Read the model definition and answer for the solid it produces. Units are mm, in the model's axes. Face numbers are marked on the shaded views. A direction names the side the tool comes from. Give positions to 0.01 mm unless a question says otherwise; leave off trailing zeros. Order: outer loops, then holes, each group sorted by start corner. A loop starts at its lowest first (then second) coordinate and runs counter-clockwise, first axis right, second up. Notation, with made-up numbers: (29.25, 23) - (33.25, 23) arc R33 ccw to (33.25, 60) - close; hole circle Ø5 at (-1.5, 16). An arc over 180 degrees is marked (long way). Write each question's results on one line, items separated by ' | '. Start each with the question number.
Q1. Find section D-D on x = -10.5. Give the vertices of the cut face in (y, z), and give its area (3 significant figures).
Q2. Find section A-A on x = 4.75. Give the vertices of the cut face in (y, z), and give its area (3 significant figures).
Q3. Find section B-B on y = 1.15. Give the vertices of the cut face in (x, z), and give its area (3 significant figures).
Q4. Find the intervals of material crossed by line 1 along X through (y, z) = (1.1, 11); line 2 along X through (y, z) = (2.6, 8.5); line 3 along X through (y, z) = (0.3, 1), in increasing order. Write a range as from..to.
Q5. A tool of negligible diameter and unlimited length cuts with its end or side. For the marked faces 4, 5 and 6, from which of +Z, -Z, +X, -X, +Y, -Y can it reach the whole face along a straight path? Write none if from no direction.
Q6. Find section C-C on z = 3.25. Give the vertices of the cut face in (x, y), and give its area (3 significant figures).
Q7. Flat-ended cylindrical pins translate along their axes: P1, Ø1.2, axis at x = 9.5, z = 0, coming from the +Y side; P2, Ø3.5, axis at x = 9.9, z = 0, coming from the -Y side; P3, Ø0.9, axis at y = 1.5, z = -10, coming from the -X side; P4, Ø3, axis at x = -9.9, z = 0, coming from the +Y side. Find the tip coordinate at first contact, or state that the pin passes through.
Q8. For a pull along X with two mould halves and no side action, classify the marked faces 1, 2 and 3 as +X half, -X half, draft (parallel to the pull), parting line (faces both ways), or undercut.
from build123d import *

# Parameters (mm, degrees)
EXTRUDE_1_DEPTH          = 3
SKETCH_2_R               = 1.25
CUT_EXTRUDE_1_DEPTH      = 18.930421077
CUT_EXTRUDE_START        = -3
SKETCH_2_3_R             = 2
CUT_EXTRUDE_2_DEPTH      = 1.5
PATTERN_CIRCULAR_1_COUNT = 4


with BuildPart() as part:
    # 草图1 → 凸台-拉伸1 (new body)
    with BuildSketch(Plane(origin=(0, 0, 0), x_dir=(1, 0, 0), z_dir=(0, 1, 0))):
        with BuildLine():
            ThreePointArc((0, 6.2), (4.384062043, 4.384062043), (6.2, 0))
            Line((6.2, 0), (6.2, 6.2))
            Line((6.2, 6.2), (0, 6.2))
        make_face()
        with BuildLine():
            Line((-6.2, 6.2), (-6.2, 1.3e-08))
            ThreePointArc((-6.2, 1.3e-08), (-4.384062039, 4.384062048), (0, 6.2))
            Line((0, 6.2), (-6.2, 6.2))
        make_face()
        with BuildLine():
            Line((-6.2, 1.3e-08), (-6.2, -6.2))
            Line((-6.2, -6.2), (0, -6.2))
            ThreePointArc((0, -6.2), (-4.384062048, -4.384062039), (-6.2, 1.3e-08))
        make_face()
        with BuildLine():
            ThreePointArc((6.2, 0), (4.384062043, -4.384062043), (0, -6.2))
            Line((0, -6.2), (6.2, -6.2))
            Line((6.2, -6.2), (6.2, 0))
        make_face()
        Polygon((0, -6.2), (-6.2, -6.2), (-6.2, -12.5), (6.2, -12.5), (6.2, -6.2), align=None)
        Polygon((6.2, 0), (6.2, -6.2), (12.5, -6.2), (12.5, 6.2), (6.2, 6.2), align=None)
        Polygon((-6.2, 12.5), (-6.2, 6.2), (0, 6.2), (6.2, 6.2), (6.2, 12.5), align=None)
        Polygon((-12.5, 6.2), (-12.5, -6.2), (-6.2, -6.2), (-6.2, 1.3e-08), (-6.2, 6.2), align=None)
    extrude(amount=EXTRUDE_1_DEPTH)

    # 草图2 → 切除-拉伸1 (cut, through all)
    with BuildSketch(Plane(origin=(0, 0, 0), x_dir=(-1, 0, 0), z_dir=(0, -1, 0))):
        with Locations(Location((-9.899494937, 0, 0), (0, 0, 90))):
            Circle(SKETCH_2_R)
    cut_extrude_1 = extrude(amount=-CUT_EXTRUDE_1_DEPTH, mode=Mode.SUBTRACT)

    # 草图2<3> → 切除-拉伸2 (cut)
    with BuildSketch(Plane(origin=(0, 0, 0), x_dir=(-1, 0, 0), z_dir=(0, -1, 0)).offset(CUT_EXTRUDE_START)):
        with Locations(Location((-9.899494937, 0, 0), (0, 0, 270))):
            Circle(SKETCH_2_3_R)
    cut_extrude_2 = extrude(amount=CUT_EXTRUDE_2_DEPTH, mode=Mode.SUBTRACT)

    # 阵列(圆周)1: 切除-拉伸1, 切除-拉伸2 ×4 about axis
    pattern_circular_1_axis = Axis((0, 0, 0), (0, 1, 0))
    add([cut_extrude_1.rotate(pattern_circular_1_axis, i * 360 / PATTERN_CIRCULAR_1_COUNT) for i in range(1, PATTERN_CIRCULAR_1_COUNT)], mode=Mode.SUBTRACT)
    add([cut_extrude_2.rotate(pattern_circular_1_axis, i * 360 / PATTERN_CIRCULAR_1_COUNT) for i in range(1, PATTERN_CIRCULAR_1_COUNT)], mode=Mode.SUBTRACT)


solid = part.part
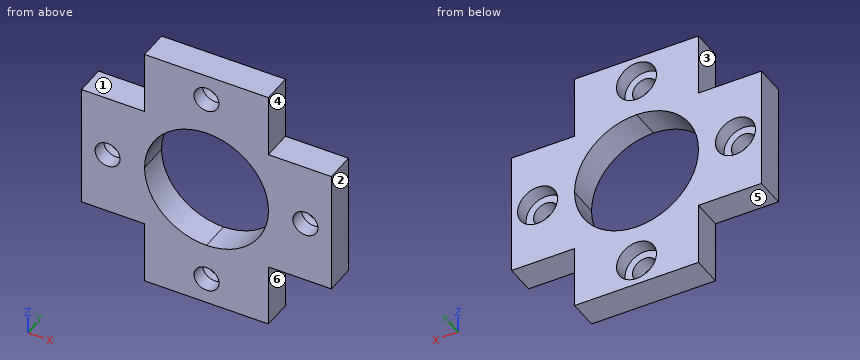
Working result:
1) outline: (0, -6.2) - (3, -6.2) - (3, -1.91) - (1.5, -1.91) - (1.5, -1.1) - (0, -1.1) - close; (0, 1.1) - (1.5, 1.1) - (1.5, 1.91) - (3, 1.91) - (3, 6.2) - (0, 6.2) - close | area: 28.2 mm²
2) outline: (0, -12.5) - (3, -12.5) - (3, -3.98) - (0, -3.98) - close; (0, 3.98) - (3, 3.98) - (3, 12.5) - (0, 12.5) - close | area: 51.1 mm²
3) outline: (-12.5, -6.2) - (-6.2, -6.2) - (-6.2, -12.5) - (6.2, -12.5) - (6.2, -6.2) - (12.5, -6.2) - (12.5, 6.2) - (6.2, 6.2) - (6.2, 12.5) - (-6.2, 12.5) - (-6.2, 6.2) - (-12.5, 6.2) - close; hole circle Ø2.5 at (-9.9, 0); hole circle Ø12.4 at (0, 0); hole circle Ø2.5 at (0, -9.9); hole circle Ø2.5 at (0, 9.9); hole circle Ø2.5 at (9.9, 0) | area: 326 mm²
4) line 1: -6.2..-0.59, 0.59..6.2 | line 2: -6.2..-1.43, 1.43..6.2 | line 3: -12.5..-10.65, -9.15..-6.12, 6.12..9.15, 10.65..12.5
5) face 4: +Z, +X, +Y, -Y | face 5: -Z, -X, +Y, -Y | face 6: -Z, +X, +Y, -Y
6) outline: (-12.5, 0) - (-5.28, 0) - (-5.28, 3) - (-12.5, 3) - close; (5.28, 0) - (12.5, 0) - (12.5, 3) - (5.28, 3) - close | area: 43.3 mm²
7) P1: through | P2: y = 0 | P3: x = -6.2 | P4: y = 1.5
8) face 1: draft | face 2: +X half | face 3: -X half
